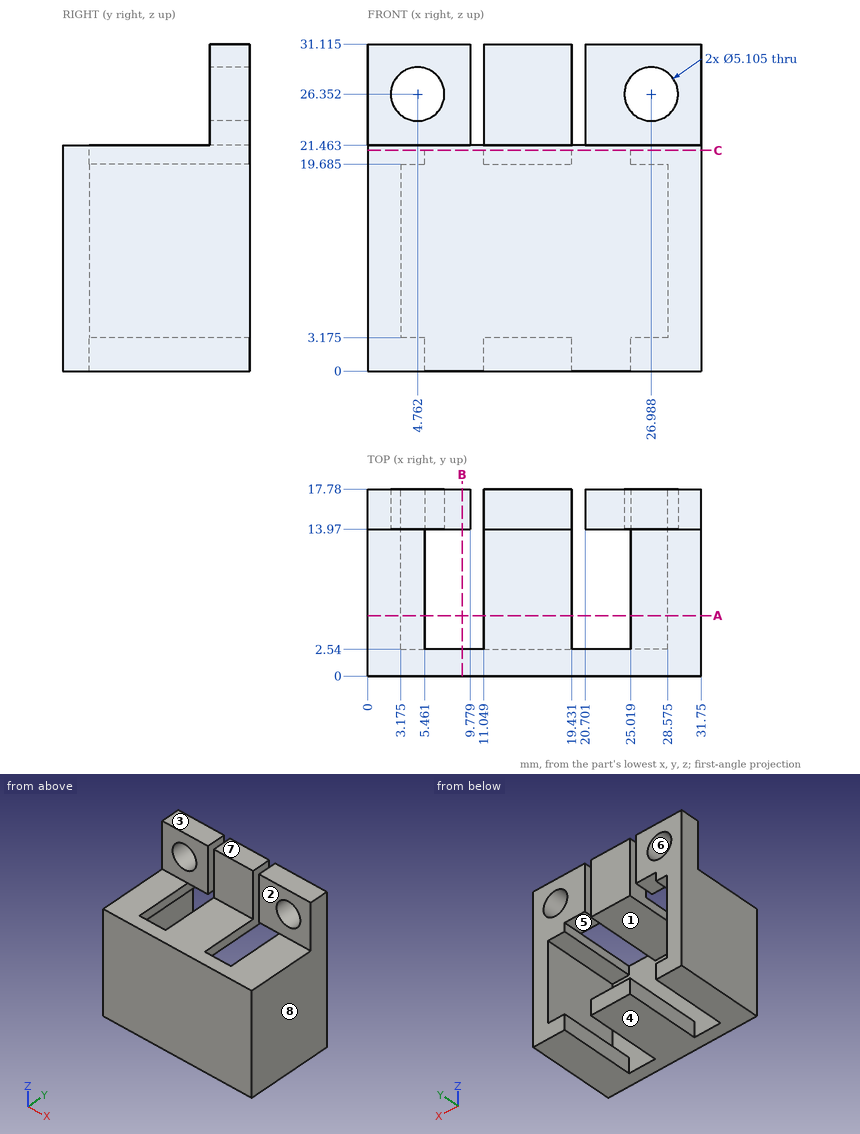
Can you work these out from the drawing? Everything is in mm from the part's minimum corner. A direction names the side the tool comes from. Coordinates: 2 decimals unless noted, no trailing zeros. Loops run counter-clockwise (first coordinate to the right, second up) from the corner with the lowest first, then second, coordinate; pieces in that order, holes last. Notation, with made-up numbers: (59.25, 7.5) - (100.25, 7.5) arc R20 ccw to (100.25, 26.5) - close; hole circle Ø2 at (82.5, -27). An arc over 180 degrees is marked (long way). Use a Markdown table: item, result.
Item 1: For the marked faces 1, 2, 3, 4 and 5, which set-ups out of +Z, -Z, +X, -X, +Y, -Y let a thin tool reach every point of the face, with its end or its side?
Numbers:
| item | result |
|---|---|
| face 1 | +Y |
| face 2 | +Z, +X, -X, -Y |
| face 3 | +Z, +X, -X, +Y, -Y |
| face 4 | -Z, +X, -X, +Y, -Y |
| face 5 | -Z, +Y |
Item 2: If I drill on probe 1 along X at (y, z) = (11.5, 1.5); probe 2 along Z at (x, y) = (4, 8.75) (1 decimal); probe 3 along Y at (x, z) = (8, 12), over which ranges is the centre line in solid material (lowest first)? Write a range as from..to.
Numbers:
| item | result |
|---|---|
| probe 1 | x = 0..5.46, 11.05..19.43, 25.02..31.75 |
| probe 2 | z = 0..3.2, 19.7..21.5 |
| probe 3 | y = 0..2.54 |
Item 3: Will these pins go through, and if not, where does the flat tip stop? pin 1 (5 mm diameter, centred on x = 22, y = 13, fed in from -Z); pin 2 (3.5 mm diameter, centred on y = 12.5, z = 2, fed in from -X); pin 3 (4 mm diameter, centred on x = 18, y = 8, fed in from +Z); pin 4 (3 mm diameter, centred on x = 6.5, z = 27.5, fed in from -Y).
Numbers:
| item | result |
|---|---|
| pin 1 | stops at z = 21.46 |
| pin 2 | stops at x = 0 |
| pin 3 | stops at z = 21.46 |
| pin 4 | stops at y = 13.97 |
Item 4: We'd pull the mould along Z, two halves only. Please class the marked faces 6, 7 and 8: released by +Z, released by -Z, zero draft, split by the parting line, or undercut.
Numbers:
| item | result |
|---|---|
| face 6 | undercut |
| face 7 | released by +Z |
| face 8 | zero draft |
Item 5: I want a section at C-C on z = 21. Please give me the cut outline in (x, y).
Numbers:
| item | result |
|---|---|
| outline | (0, 0) - (31.75, 0) - (31.75, 17.78) - (25.02, 17.78) - (25.02, 2.54) - (19.43, 2.54) - (19.43, 17.78) - (11.05, 17.78) - (11.05, 2.54) - (5.46, 2.54) - (5.46, 17.78) - (0, 17.78) - close |
Item 6: I want a section at A-A on y = 5.75. Give the number of separate pieces and of enclosed holes in the cut face, and give its area (3 significant figures).
Numbers:
| item | result |
|---|---|
| separate pieces | 4 |
| enclosed holes | 0 |
| area | 207 mm2 |
Item 7: I want a section at B-B on x = 9. Please give me the cut outline in (y, z) (1 decimal).
Numbers:
| item | result |
|---|---|
| outline | (0, 0) - (2.5, 0) - (2.5, 21.5) - (0, 21.5) - close; (14, 21.5) - (17.8, 21.5) - (17.8, 31.1) - (14, 31.1) - close |
